```python
from build123d import *

# Parameters (mm, degrees)
ESQUISSE1_R        = 1.5
BOSS_EXTRU_1_DEPTH = 5


with BuildPart() as part:
    # Esquisse1 → Boss.-Extru.1 (new body)
    with BuildSketch(Plane.XY):
        Polygon((-25, 81.290322581), (15, 81.290322581), (15, 76.290322581), (75, 76.290322581), (75, 81.290322581), (115, 81.290322581), (115, 51.290322581), (110, 51.290322581), (110, 23.790322581), (100, 23.790322581), (100, 26.290322581), (95, 26.290322581), (95, 23.790322581), (90, 23.790322581), (90, 18.790322581), (95, 18.790322581), (95, 16.290322581), (100, 16.290322581), (100, 18.790322581), (110, 18.790322581), (110, -8.709677419), (115, -8.709677419), (115, -38.709677419), (110, -38.709677419), (110, -98.709677419), (115, -98.709677419), (115, -128.709677419), (75, -128.709677419), (75, -123.709677419), (47.5, -123.709677419), (47.5, -113.709677419), (50, -113.709677419), (50, -108.709677419), (47.5, -108.709677419), (47.5, -103.709677419), (42.5, -103.709677419), (42.5, -108.709677419), (40, -108.709677419), (40, -113.709677419), (42.5, -113.709677419), (42.5, -123.709677419), (15, -123.709677419), (15, -128.709677419), (-25, -128.709677419), (-25, -123.709677419), (-85, -123.709677419), (-85, -128.709677419), (-125, -128.709677419), (-125, -98.709677419), (-120, -98.709677419), (-120, -71.209677419), (-110, -71.209677419), (-110, -73.709677419), (-105, -73.709677419), (-105, -71.209677419), (-100, -71.209677419), (-100, -66.209677419), (-105, -66.209677419), (-105, -63.709677419), (-110, -63.709677419), (-110, -66.209677419), (-120, -66.209677419), (-120, -38.709677419), (-125, -38.709677419), (-125, -8.709677419), (-120, -8.709677419), (-120, 51.290322581), (-125, 51.290322581), (-125, 81.290322581), (-85, 81.290322581), (-85, 76.290322581), (-57.5, 76.290322581), (-57.5, 66.290322581), (-60, 66.290322581), (-60, 61.290322581), (-57.5, 61.290322581), (-57.5, 56.290322581), (-52.5, 56.290322581), (-52.5, 61.290322581), (-50, 61.290322581), (-50, 66.290322581), (-52.5, 66.290322581), (-52.5, 76.290322581), (-25, 76.290322581), align=None)
        with Locations((-114.5, -93.209677419)):
            Circle(ESQUISSE1_R, mode=Mode.SUBTRACT)
        with Locations((-114.5, -115.209677419)):
            Circle(ESQUISSE1_R, mode=Mode.SUBTRACT)
        with Locations((-87.5, -115.209677419)):
            Circle(ESQUISSE1_R, mode=Mode.SUBTRACT)
        with Locations((-87.5, -93.209677419)):
            Circle(ESQUISSE1_R, mode=Mode.SUBTRACT)
        with Locations(Location((-87.5, 45.790322581, 0), (0, 0, 180))):
            Circle(ESQUISSE1_R, mode=Mode.SUBTRACT)
        with Locations(Location((-87.5, 67.790322581, 0), (0, 0, 180))):
            Circle(ESQUISSE1_R, mode=Mode.SUBTRACT)
        with Locations(Location((-114.5, 67.790322581, 0), (0, 0, 180))):
            Circle(ESQUISSE1_R, mode=Mode.SUBTRACT)
        with Locations(Location((-114.5, 45.790322581, 0), (0, 0, 180))):
            Circle(ESQUISSE1_R, mode=Mode.SUBTRACT)
        with Locations((104.5, 67.790322581)):
            Circle(ESQUISSE1_R, mode=Mode.SUBTRACT)
        with Locations((104.5, 45.790322581)):
            Circle(ESQUISSE1_R, mode=Mode.SUBTRACT)
        with Locations((77.5, 45.790322581)):
            Circle(ESQUISSE1_R, mode=Mode.SUBTRACT)
        with Locations((77.5, 67.790322581)):
            Circle(ESQUISSE1_R, mode=Mode.SUBTRACT)
        with Locations(Location((104.5, -93.209677419, 0), (0, 0, 180))):
            Circle(ESQUISSE1_R, mode=Mode.SUBTRACT)
        with Locations(Location((104.5, -115.209677419, 0), (0, 0, 180))):
            Circle(ESQUISSE1_R, mode=Mode.SUBTRACT)
        with Locations(Location((77.5, -115.209677419, 0), (0, 0, 180))):
            Circle(ESQUISSE1_R, mode=Mode.SUBTRACT)
        with Locations(Location((77.5, -93.209677419, 0), (0, 0, 180))):
            Circle(ESQUISSE1_R, mode=Mode.SUBTRACT)
    extrude(amount=BOSS_EXTRU_1_DEPTH)


solid = part.part
```
Model file for the job. Use its own axes, mm. A direction names the side the tool comes from. Give positions to 0.01 mm unless a question says otherwise; leave off trailing zeros. Loops run counter-clockwise (first coordinate to the right, second up) from the corner with the lowest first, then second, coordinate; pieces in that order, holes last. Notation, with made-up numbers: (19.5, 51) -> (33.5, 51) arc R20 ccw to (33.5, 63) -> close; hole circle Ø3 at (65.5, 45). An arc over 180 degrees is marked (long way). Use CSV: the item, a comma, the result in double quotes. Start each with the question number.
1) Slice it at C-C on z = 3.9. Give the number of separate pieces and of enclosed holes in the cut face, plus the area to 3 significant figures.
2) Tool access for faces 4 (the flat face through (-52.5, 59, 2)), 5 (the flat face through (92, 18.79, 2)), 6 (the flat face through (97, 16.29, 2)), 7 (the flat face through (47.5, -119, 2)): list every direction of +Z, -Z, +X, -X, +Y, -Y with a clear straight run to the whole face (end or side of a thin tool).
3) Mould opens along X. For faces 1 (the flat face through (-125, -114, 2)), 2 (the flat face through (15, -126, 2)), 3 (the flat face through (110, 5, 2)) say: released by +X, released by -X, zero draft, split by the parting line, or undercut.
4) Slice it at B-B on x = -41.5. Give the cut face in (y, z).
5) Slice it at A-A on y = -54. Give the cut face in (x, z).
6) Flat gauge pins, fed straight in: pin 1 Ø2.5 at (x, z) = (61.5, 3.5) entering from -Y; pin 2 Ø1.5 at (x, z) = (-30, 2.5) entering from +Y; pin 3 Ø1.5 at (y, z) = (-83, 1.5) entering from +X. Where does each tip first touch, or does it go through?
7) Wall check: line 1 (Y direction, x = 104.5, z = 1.05); line 2 (Y direction, x = 77.5, z = 3.7); line 3 (Y direction, x = -114.5, z = 1.85). Give the ranges that are in metal, low to high.
Computed values:
1,separate pieces,"1"
1,enclosed holes,"16"
1,area,"47,400 mm^2"
2,face 4,"+Z, -Z, +Y"
2,face 5,"+Z, -Z, +X"
2,face 6,"+Z, -Z"
2,face 7,"+Z, -Z, -Y"
3,face 1,"released by -X"
3,face 2,"undercut"
3,face 3,"released by +X"
4,outline,"(-123.71, 0) -> (76.29, 0) -> (76.29, 5) -> (-123.71, 5) -> close"
5,outline,"(-120, 0) -> (110, 0) -> (110, 5) -> (-120, 5) -> close"
6,pin 1,"stops at y = -123.71"
6,pin 2,"stops at y = 76.29"
6,pin 3,"stops at x = 110"
7,line 1,"y = -128.71 to -116.71, -113.71 to -94.71, -91.71 to 18.79, 23.79 to 44.29, 47.29 to 66.29, 69.29 to 81.29"
7,line 2,"y = -128.71 to -116.71, -113.71 to -94.71, -91.71 to 44.29, 47.29 to 66.29, 69.29 to 81.29"
7,line 3,"y = -128.71 to -116.71, -113.71 to -94.71, -91.71 to -71.21, -66.21 to 44.29, 47.29 to 66.29, 69.29 to 81.29"
